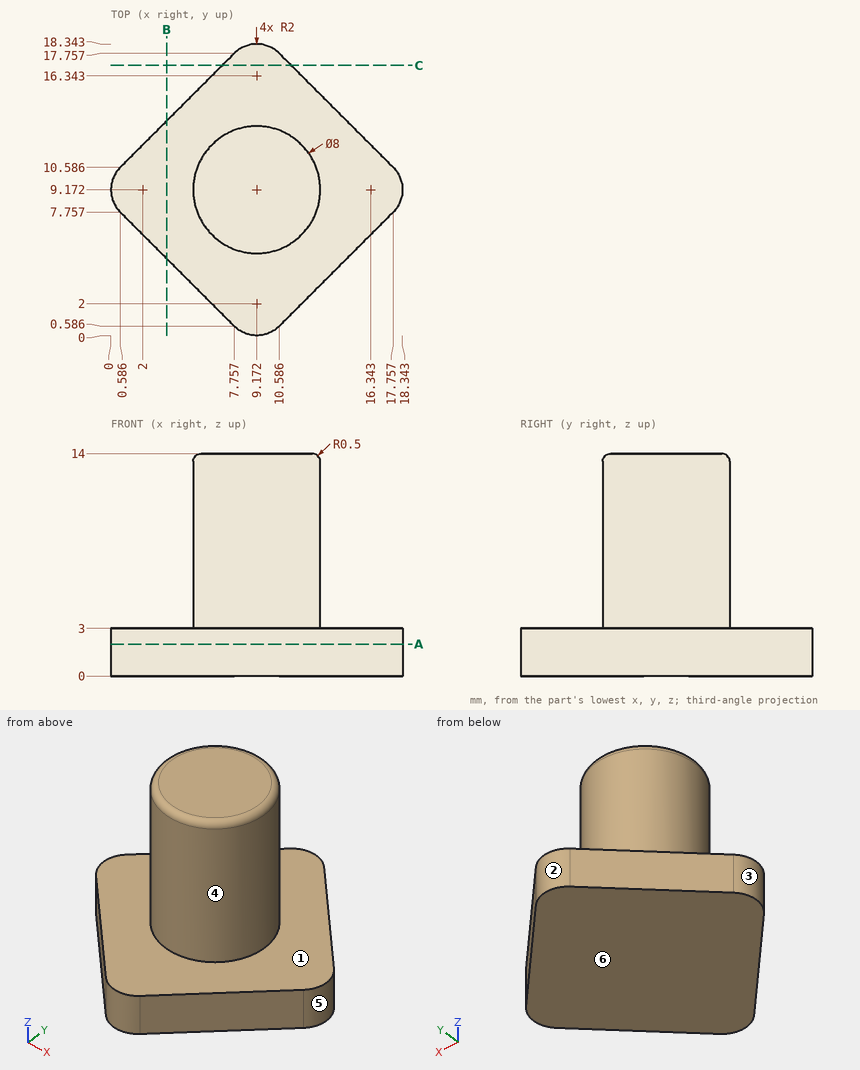
Study the drawing (mm; zero at the part's minimum x, y, z) and answer. A direction names the side the tool comes from. Give positions to 0.01 mm unless a question says otherwise; leave off trailing zeros. Loops run counter-clockwise (first coordinate to the right, second up) from the corner with the lowest first, then second, coordinate; pieces in that order, holes last. Notation, with made-up numbers: M -33,-3 L -1,-3 A8 ccw -1,9 Z; hole C 78,53 d3. An arc over 180 degrees is marked long. One line per item, written item: value. Start each with the question number.
1. Which of the six approach directions +Z, -Z, +X, -X, +Y, -Y give full straight-line access (tool end or side, diameter ignored) to the marked faces 1 and 2?
2. Find section C-C (y = 17). Give the vertices of the cut face in (x, z), and give its area (3 significant figures).
3. Find section A-A (z = 2). Give the vertices of the cut face in (x, y) (1 decimal), and give its area (3 significant figures).
4. Find section B-B (x = 3.5). Give the vertices of the cut face in (y, z), and give its area (3 significant figures).
5. Each of these flat-tipped pins is pushed along its axis until it touches: P1, Ø2, axis at x = 13, y = 4.5, coming from the +Z side; P2, Ø1.5, axis at y = 13.5, z = 4.5, coming from the -X side (1 decimal); P3, Ø4, axis at y = 3.5, z = 7, coming from the +X side. Where does it stop, or does it pass through?
6. Find the intervals of material crossed by probe 1 along Z at (x, y) = (1.5, 10.5); probe 2 along Y at (x, z) = (9.5, 9.75) (1 decimal); probe 3 along X at (y, z) = (7.25, 9.5) (1 decimal), in increasing order.
7. Determine the mould class of the marked faces 3, 4, 5 and 6 for opening direction X: released by +X, released by -X, zero draft, split by the parting line, or undercut.
Reported:
1. face 1: +Z
1. face 2: +Z, -Z, +Y
2. outline: M 7,0 L 11.34,0 L 11.34,3 L 7,3 Z
2. area: 13.0 mm²
3. outline: M 0.6,7.8 L 7.8,0.6 A2 ccw 10.6,0.6 L 17.8,7.8 A2 ccw 17.8,10.6 L 10.6,17.8 A2 ccw 7.8,17.8 L 0.6,10.6 A2 ccw Z
3. area: 197 mm²
4. outline: M 4.84,0 L 13.5,0 L 13.5,3 L 4.84,3 Z
4. area: 26.0 mm²
5. P1: stops at z = 3
5. P2: stops at x = 7.4
5. P3: stops at x = 10.76
6. probe 1: z = 0 to 3
6. probe 2: y = 5.2 to 13.2
6. probe 3: x = 5.7 to 12.7
7. face 3: released by -X
7. face 4: split by the parting line
7. face 5: released by +X
7. face 6: zero draft
